Verification items for the finished model (mm, model axes). Face numbers are marked on the shaded views. A direction names the side the tool comes from. Give positions to 0.01 mm unless a question says otherwise; leave off trailing zeros. Order: outer loops, then holes, each group sorted by start corner. A loop starts at its lowest first (then second) coordinate and runs counter-clockwise, first axis right, second up. Notation, with made-up numbers: (45.5, 10) -> (90.5, 10) arc R17 ccw to (90.5, 39) -> close; hole circle Ø9 at (63.5, 58). An arc over 180 degrees is marked (long way). One line per question, with ' | ' between items. Start each with the question number.
Q1. Access from +Z, -Z, +X, -X, +Y, -Y to the whole of each face (thin tool, end or side, straight path). Record for the marked faces 1, 2 and 3.
Q2. Material ranges on probe 1 along X at (y, z) = (1.1, 6.75); probe 2 along Y at (x, z) = (0, 8.5); probe 3 along Z at (x, y) = (-25, 0.7), recorded low to high. Write a range as [from, to].
Q3. Section check D-D on x = 0. Record the cut outline in (y, z), plus the area to 3 significant figures.
Q4. Mould release check, pull along Y, two halves, no side actions. Record for the marked faces 4, 5 and 6: released by +Y, released by -Y, zero draft, split by the parting line, or undercut.
Q5. Section check A-A on x = -25. Record the cut outline in (y, z).
Q6. Section check B-B on z = 6.75. Record the cut outline in (x, y).
Q7. Section check C-C on y = 14. Record the cut outline in (x, z).
Q8. Go/stop test with flat-tipped pins: pin 1 (4.5 mm diameter, centred on x = -25, z = 6.75, fed in from +Y); pin 2 (8 mm diameter, centred on y = 10, z = 7.5, fed in from -X); pin 3 (5.5 mm diameter, centred on x = 25, z = 6.75, fed in from +Y). Record where each tip stops, or that it passes through.
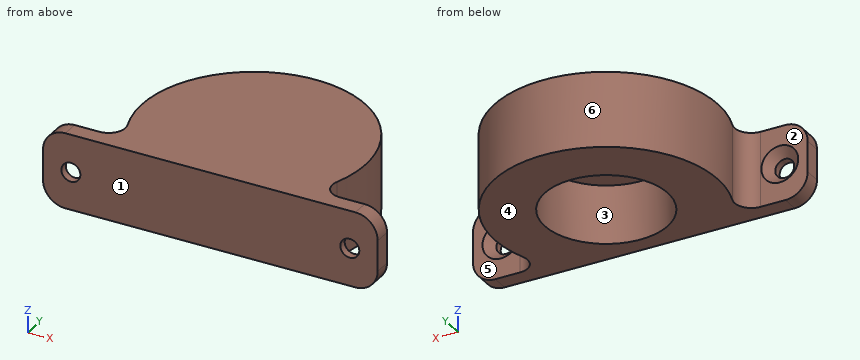
Autodesk Inventor part; units mm, degrees
ref_plane "YZ Plane" through (0, 0, 0) normal (1, 0, 0) x (0, 1, 0)
ref_plane "XZ Plane" through (0, 0, 0) normal (0, 1, 0) x (-1, 0, 0)
ref_plane "XY Plane" through (0, 0, 0) normal (0, 0, 1) x (1, 0, 0)
sketch "Эскиз1" plane through (0, 0, 0) normal (0, 0, 1) x (1, 0, 0)
  line L0 (-30, 0) -> (30, 0)
  line L1 (-30, 0) -> (-30, 3)
  line L2 (-30, 3) -> (-16.7033, 3)
  line L3 (16.7033, 3) -> (30, 3)
  line L4 (30, 3) -> (30, 0)
  line L5 (0, 0) -> (0, -12) construction
  circle A0 centre (0, 14) radius 11 construction
  circle A1 centre (0, 14) radius 11
  arc A2 (16.7033, 3) -> (-16.7033, 3) centre (0, 14) ccw
  point P0 (0, 3)
  point P1 (0, 46)
  point P2 (0, 25)
  dimension "d3" = 3
  dimension "d8" = 22
  dimension "d9" = 14
  dimension "d25" = 40
  dimension "d39" = 30
extrude "Выдавливание1" add sketch "Эскиз1" along normal blind 10.5
sketch "Эскиз2" plane through (0, 0, 10.5) normal (0, 0, 1) x (1, 0, 0)
  line L0 (-30, 0) -> (30, 0)
  line L1 (30, 0) -> (30, 3)
  line L2 (30, 3) -> (16.7033, 3)
  line L3 (-16.7033, 3) -> (-30, 3)
  line L4 (-30, 3) -> (-30, 0)
  circle A0 centre (0, 14) radius 11
  arc A1 (16.7033, 3) -> (-16.7033, 3) centre (0, 14) ccw
  point P0 (0, 0)
extrude "Выдавливание2" add sketch "Эскиз2" along normal blind 3 contours L4 L3 A1 L2 L1 L0 | A0
fillet "Сопряжение1" radius 4 4 edges at (30, 1.5, 0) (30, 1.5, 13.5) (-30, 1.5, 0) (-30, 1.5, 13.5)
fillet "Сопряжение1" radius 3 2 edges at (16.7033, 3, 6.75) (-16.7033, 3, 6.75)
sketch "Эскиз4" plane through (21.5639, 3, 0) normal (0, 1, 0) x (1, 0, 0)
  line L0 (-43.1277, 0) -> (-43.1277, -13.5)
  line L1 (-43.1277, 0) -> (-47.5639, 0)
  arc A0 (-47.5639, 0) -> (-51.5639, -4) centre (-47.5639, -4) ccw
  line L2 (-51.5639, -4) -> (-51.5639, -9.5)
  arc A1 (-51.5639, -9.5) -> (-47.5639, -13.5) centre (-47.5639, -9.5) ccw
  line L3 (-43.1277, -13.5) -> (-47.5639, -13.5)
  point P0 (-21.5639, 0)
  point P1 (-46.5639, -6.75)
  dimension "d29" = 5
  dimension "d30" = 6.75
hole "Отверстие2" at (-25, 3, 6.75) direction (0, -1, 0) diameter 3.4 depth 3.7 countersink diameter 6.6 countersink angle 90
mirror "Зеркальное отражение2" about plane through (0, 0, 0) normal (1, 0, 0) of "Отверстие2"
properties part number "корпус подшипник"
Filled in:
1) face 1: +Z, -Z, +X, -X, -Y | face 2: +Z, -Z, -X, +Y | face 3: -Z
2) probe 1: [-30, -26.7], [-23.3, 23.3], [26.7, 30] | probe 2: [0, 3], [25, 34] | probe 3: [0, 5.05], [8.45, 13.5]
3) outline: (0, 0) -> (3, 0) -> (3, 10.5) -> (25, 10.5) -> (25, 0) -> (34, 0) -> (34, 13.5) -> (0, 13.5) -> close | area: 228 mm²
4) face 4: zero draft | face 5: released by +Y | face 6: undercut
5) outline: (0, 0) -> (3, 0) -> (3, 3.45) -> (1.4, 5.05) -> (0, 5.05) -> close; (0, 8.45) -> (1.4, 8.45) -> (3, 10.05) -> (3, 13.5) -> (0, 13.5) -> close
6) outline: (-30, 0) -> (-26.7, 0) -> (-26.7, 1.4) -> (-28.3, 3) -> (-30, 3) -> close; (-23.3, 0) -> (23.3, 0) -> (23.3, 1.4) -> (21.7, 3) -> (21.56, 3) arc R3 cw to (18.75, 7.04) arc R20 ccw (long way) to (-18.75, 7.04) arc R3 cw to (-21.56, 3) -> (-21.7, 3) -> (-23.3, 1.4) -> close; (26.7, 0) -> (30, 0) -> (30, 3) -> (28.3, 3) -> (26.7, 1.4) -> close; hole circle Ø22 at (0, 14)
7) outline: (-20, 0) -> (-11, 0) -> (-11, 10.5) -> (11, 10.5) -> (11, 0) -> (20, 0) -> (20, 13.5) -> (-20, 13.5) -> close
8) pin 1: y = 1.95 | pin 2: x = -20 | pin 3: y = 2.45
